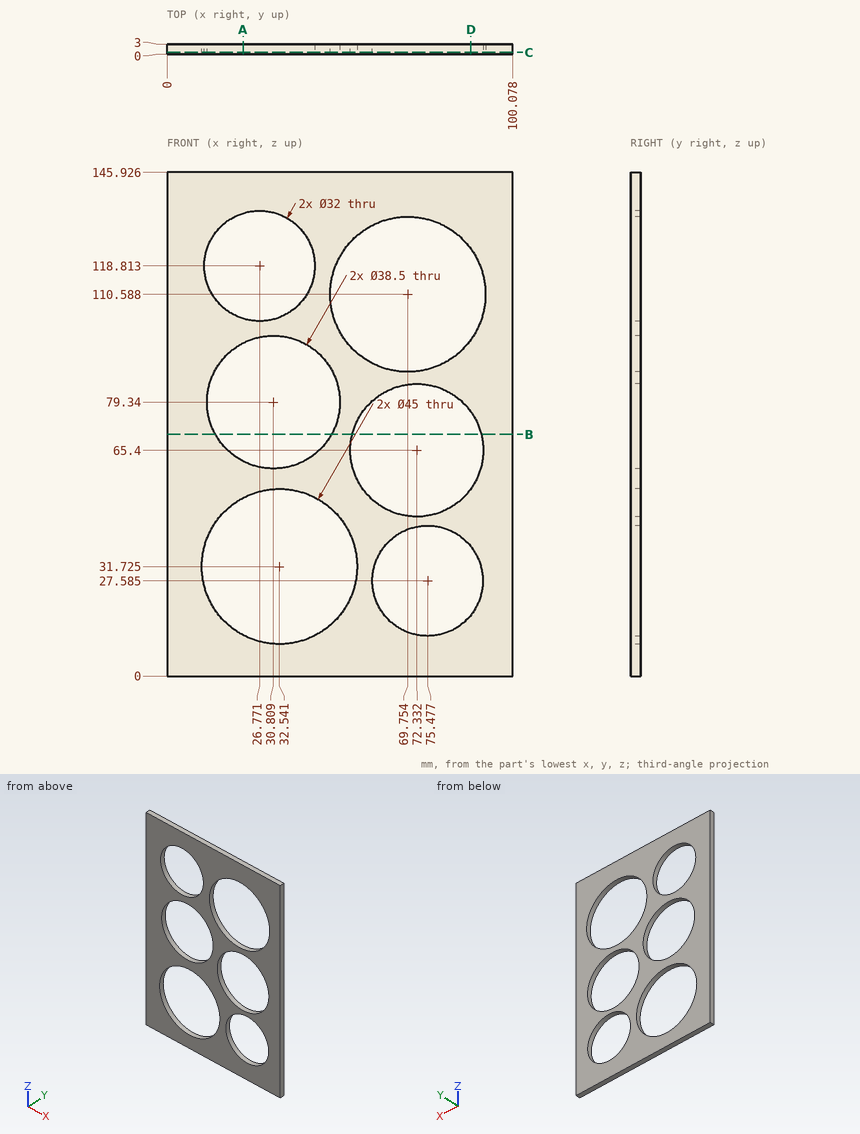
Can you work these out from the drawing? Everything is in mm from the part's minimum corner. Give positions to 0.01 mm unless a question says otherwise; leave off trailing zeros. Loops run counter-clockwise (first coordinate to the right, second up) from the corner with the lowest first, then second, coordinate; pieces in that order, holes last. Notation, with made-up numbers: M 2,64.25 L 25,64.25 A23 cw 25,76.25 Z; hole C 34,-3 d7. An arc over 180 degrees is marked long. Use CSV: the item, a comma, the result in double quotes. Start each with the question number.
1. If I drill on L1, parallel to X at y = 1.4, z = 73 (1 decimal); L2, parallel to Z at x = 71.5, y = 1.5 (1 decimal); L3, parallel to Z at x = 76, y = 2 (1 decimal), over which ranges is the centre line in solid material (lowest first)?
2. Imagine slicing it at C-C, the plane y = 0.55. Count the separate pieces of the cut face and the enclosed holes in it, plus the area to 3 significant figures.
3. Imagine slicing it at A-A, the plane x = 22. Write out the boundary of the cut face in (y, z) (1 decimal), plus the area to 3 significant figures.
4. Imagine slicing it at B-B, the plane z = 70. Write out the boundary of the cut face in (x, y) (1 decimal).
5. Imagine slicing it at D-D, the plane x = 88. Write out the boundary of the cut face in (y, z) (1 decimal).
Response values:
1,L1,"0 to 12.6, 49 to 54.6, 90 to 100.1"
1,L2,"0 to 12.1, 43.1 to 46.2, 84.6 to 88.2, 133 to 145.9"
1,L3,"0 to 11.6, 43.6 to 46.5, 84.3 to 89, 132.2 to 145.9"
2,separate pieces,"1"
2,enclosed holes,"6"
2,area,"7,490 mm^2"
3,outline,"M 0,0 L 3,0 L 3,11.8 L 0,11.8 Z; M 0,51.6 L 3,51.6 L 3,62.2 L 0,62.2 Z; M 0,96.5 L 3,96.5 L 3,103.5 L 0,103.5 Z; M 0,134.1 L 3,134.1 L 3,145.9 L 0,145.9 Z"
3,area,"124 mm^2"
4,outline,"M 0,0 L 14,0 L 14,3 L 0,3 Z; M 47.6,0 L 53.6,0 L 53.6,3 L 47.6,3 Z; M 91,0 L 100.1,0 L 100.1,3 L 91,3 Z"
5,outline,"M 0,0 L 3,0 L 3,17.6 L 0,17.6 Z; M 0,37.5 L 3,37.5 L 3,54.2 L 0,54.2 Z; M 0,76.6 L 3,76.6 L 3,97.4 L 0,97.4 Z; M 0,123.8 L 3,123.8 L 3,145.9 L 0,145.9 Z"
